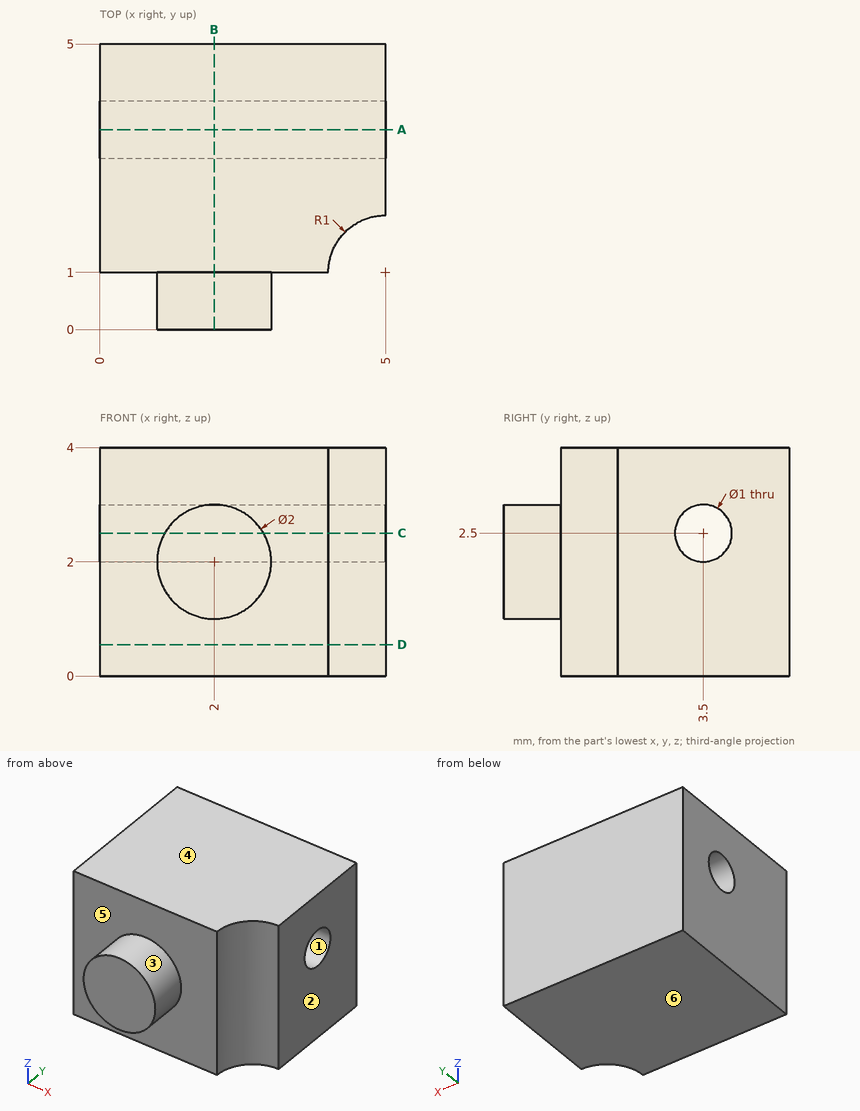
Print and shaded views of the part. All mm, measured from the part's lowest x, y and z. A direction names the side the tool comes from. Give positions to 0.01 mm unless a question says otherwise; leave off trailing zeros. Loops run counter-clockwise (first coordinate to the right, second up) from the corner with the lowest first, then second, coordinate; pieces in that order, holes last. Notation, with made-up numbers: (24.5, 45.5) -> (43.5, 45.5) arc R25 cw to (43.5, 63.5) -> close; hole circle Ø1 at (62, -12). An arc over 180 degrees is marked (long way). Use a Markdown table: item, result.
1. Slice it at D-D (z = 0.55). List the corners of the cut face in (x, y), plus the area to 3 significant figures.
Check result:
| item | result |
|---|---|
| outline | (0, 1) -> (4, 1) arc R1 cw to (5, 2) -> (5, 5) -> (0, 5) -> close |
| area | 19.2 mm^2 |
2. Wall check: L1, parallel to Z at x = 3.4, y = 3.5; L2, parallel to Y at x = 2.05, z = 0.7; L3, parallel to Y at x = 2.7, z = 2.8. Give the ranges that are in metal, low to high. Write a range as [from, to].
Check result:
| item | result |
|---|---|
| L1 | z = [0, 2], [3, 4] |
| L2 | y = [1, 5] |
| L3 | y = [1, 3.1], [3.9, 5] |
3. Which spindle directions (+Z, -Z, +X, -X, +Y, -Y) get a long thin tool onto all of the face, cutting with end or side? Do the marked faces 5 and 6. Say none if no direction does.
Check result:
| item | result |
|---|---|
| face 5 | -Y |
| face 6 | -Z, +X, -X, +Y, -Y |
4. Flat gauge pin, fed straight in: pin 1 (1 mm diameter, centred on y = 1, z = 2, fed in from +X). Where does the tip first touch, or does it go through?
Check result:
| item | result |
|---|---|
| pin 1 | stops at x = 4.13 |
5. Slice it at A-A (y = 3.5). List the corners of the cut face in (x, z), plus the area to 3 significant figures.
Check result:
| item | result |
|---|---|
| outline | (0, 0) -> (5, 0) -> (5, 2) -> (0, 2) -> close; (0, 3) -> (5, 3) -> (5, 4) -> (0, 4) -> close |
| area | 15.0 mm^2 |
6. Mould opens along Z. For the marked faces 1, 2, 3 and 4 say: pulls with the +Z half, pulls with the -Z half, needs draft (parallel to the pull), parting line crosses it, or undercut.
Check result:
| item | result |
|---|---|
| face 1 | undercut |
| face 2 | needs draft |
| face 3 | parting line crosses it |
| face 4 | pulls with the +Z half |
7. Slice it at C-C (z = 2.5). List the corners of the cut face in (x, y).
Check result:
| item | result |
|---|---|
| outline | (0, 1) -> (1.13, 1) -> (1.13, 0) -> (2.87, 0) -> (2.87, 1) -> (4, 1) arc R1 cw to (5, 2) -> (5, 3) -> (0, 3) -> close; (0, 4) -> (5, 4) -> (5, 5) -> (0, 5) -> close |
8. Slice it at B-B (x = 2). List the corners of the cut face in (y, z).
Check result:
| item | result |
|---|---|
| outline | (0, 1) -> (1, 1) -> (1, 0) -> (5, 0) -> (5, 4) -> (1, 4) -> (1, 3) -> (0, 3) -> close; hole circle Ø1 at (3.5, 2.5) |
